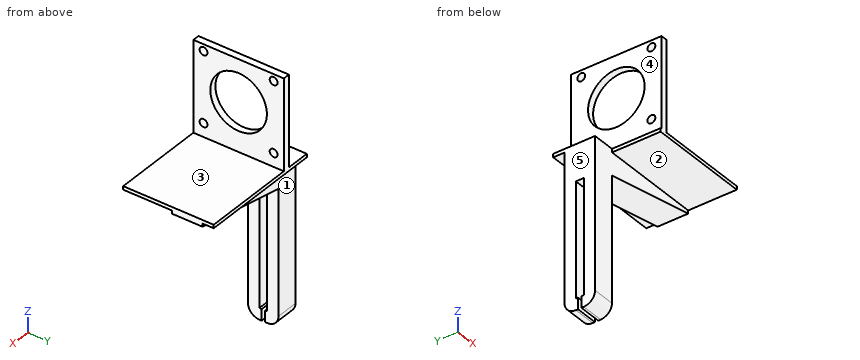
```python
from build123d import *

# Parameters (mm, degrees)
F1_DEPTH      = 10
F2_W          = 1.5
F2_H          = 5
F3_DEPTH      = 11
F4_W          = 3
F4_H          = 40
F5_DEPTH      = 35
F5_DEPTH_BACK = 5
F6_W          = 13.5
F6_H          = 10
F7_DEPTH      = 45
F9_DEPTH      = 15
F10_R         = 1.75
F10_R_2       = 12.5
F11_DEPTH     = 25
F12_W         = 10
F12_H         = 21.5
F13_DEPTH     = 25


with BuildPart() as f1:
    # F0 (on Right) → F1 (new body)
    with BuildSketch(Plane.YZ):
        with BuildLine():
            Line((-8.5, 0), (-5, 0))
            ThreePointArc((-5, 0), (-1.464466, 1.464466), (0, 5))
            Line((0, 5), (0, 70))
            Line((0, 70), (-13.5, 70))
            Line((-13.5, 70), (-13.5, 5))
            ThreePointArc((-13.5, 5), (-12.035534, 1.464466), (-8.5, 0))
        make_face()
    extrude(amount=F1_DEPTH)

    # F2 (on face) → F3 (cut)
    with BuildSketch(Plane.YZ.offset(10)):
        Polygon((-5, 55.5), (-8.5, 55.5), (-8.5, 5), (-7.441577, 5), (-5.941577, 5), (-5, 5), align=None)
        with Locations((-6.691577, 2.5)):
            Rectangle(F2_W, F2_H)
    extrude(amount=-F3_DEPTH, mode=Mode.SUBTRACT)

    # F4 (on Front) → F5 (join, two sides)
    with BuildSketch(Plane.XZ) as f5_sk:
        Polygon((10.552509, 71.532604), (0, 71.532604), (0, 70), (55, 70), (55, 71.532604), (13.552509, 71.532604), align=None)
        with Locations((12.052509, 91.532604)):
            Rectangle(F4_W, F4_H)
    extrude(amount=F5_DEPTH)
    extrude(f5_sk.sketch, amount=-F5_DEPTH_BACK)

    # F6 (on face) → F7 (join, through all)
    with BuildSketch(Plane.YZ.offset(10)):
        with Locations((-6.75, 65)):
            Rectangle(F6_W, F6_H)
    extrude(amount=F7_DEPTH)

    # F8 (on face) → F9 (cut)
    with BuildSketch(Plane.XZ.offset(13.5)):
        Polygon((55, 68.611123), (10, 60), (55, 60), align=None)
    extrude(amount=-F9_DEPTH, mode=Mode.SUBTRACT)

    # F10 (on face) → F11 (cut)
    with BuildSketch(Plane(origin=(10.552509, 0, 0), x_dir=(0, -1, 0), z_dir=(-1, 0, 0))):
        with Locations((-0.5, 108.532604)):
            Circle(F10_R)
        with Locations((30.5, 108.532604)):
            Circle(F10_R)
        with Locations((30.5, 77.532604)):
            Circle(F10_R)
        with Locations((-0.5, 77.532604)):
            Circle(F10_R)
        with Locations((15, 93.032604)):
            Circle(F10_R_2)
    extrude(amount=-F11_DEPTH, mode=Mode.SUBTRACT)

    # F12 (on face) → F13 (cut)
    with BuildSketch(Plane.XY.offset(71.532604)):
        with Locations((5, -24.25)):
            Rectangle(F12_W, F12_H)
    extrude(amount=-F13_DEPTH, mode=Mode.SUBTRACT)


solid = f1.part
```
Check sheet for the modelled part. Datum: model origin and axes. Units: mm. Face numbers are marked on the shaded views. A direction names the side the tool comes from. Give positions to 0.01 mm unless a question says otherwise; leave off trailing zeros. Write each loop counter-clockwise with the first axis right and the second up, starting at its lowest first coordinate (ties: lowest second). Pieces come first, ordered by that corner, then holes. Notation, with made-up numbers: (11, -12) -> (18, -12) arc R27 cw to (18, 21) -> close; hole circle Ø1 at (72, 6). An arc over 180 degrees is marked (long way). Use CSV: the item, a comma, the result in double quotes. Start each with the question number.
Q1. Tool access check on the marked faces 1, 2, 3, 4 and 5. Record the directions out of +Z, -Z, +X, -X, +Y, -Y that give a thin tool (end or side, any length) a straight path to the whole face; none if there is none.
Q2. Cross-section at B-B on z = 29. Enter the section's corners in (x, y), and give its area (3 significant figures).
Q3. Cross-section at D-D on x = 4.5. Enter the section's corners in (y, z).
Q4. Cross-section at A-A on y = -15. Enter the section's corners in (x, z).
Q5. Depth check by flat-ended pin: P1, Ø3, axis at x = 29, y = -5, coming from the +Z side; P2, Ø3, axis at y = -30.5, z = 77.53, coming from the +X side; P3, Ø1.2, axis at y = -22, z = 71, coming from the -X side; P4, Ø2.5, axis at x = 5, z = 3, coming from the -Y side. Enter the tip coordinate at first touch or a pass-through.
Q6. Scan lines: line 1 along Z through (x, y) = (12.1, -30.5); line 2 along Z through (x, y) = (11, -30); line 3 along Z through (x, y) = (15, -18). Record each from-to range of solid material in increasing order.
Q7. Cross-section at C-C on y = -30.5. Enter the section's corners in (x, z), and give its area (3 significant figures).
Working result:
1,face 1,"-Z, +X, -X, +Y"
1,face 2,"-Z, +X, -X, -Y"
1,face 3,"+Z, +X, +Y, -Y"
1,face 4,"+Z, -X, +Y, -Y"
1,face 5,"+Z, -Z, -X, +Y, -Y"
2,outline,"(0, -13.5) -> (10, -13.5) -> (10, -8.5) -> (0, -8.5) -> close; (0, -5) -> (10, -5) -> (10, 0) -> (0, 0) -> close"
2,area,"100 mm^2"
3,outline,"(-13.5, 5) arc R5 ccw to (-8.5, 0) -> (-7.44, 0) -> (-7.44, 5) -> (-8.5, 5) -> (-8.5, 55.5) -> (-5, 55.5) -> (-5, 5) -> (-5.94, 5) -> (-5.94, 0) -> (-5, 0) arc R5 ccw to (0, 5) -> (0, 70) -> (5, 70) -> (5, 71.53) -> (-13.5, 71.53) -> close"
4,outline,"(10, 70) -> (55, 70) -> (55, 71.53) -> (13.55, 71.53) -> (13.55, 80.53) -> (10.55, 80.53) -> (10.55, 71.53) -> (10, 71.53) -> close; (10.55, 105.53) -> (13.55, 105.53) -> (13.55, 111.53) -> (10.55, 111.53) -> close"
5,P1,"stops at z = 71.53"
5,P2,"passes through"
5,P3,"stops at x = 10"
5,P4,"stops at y = -13.44"
6,line 1,"z = 70 to 75.78, 79.28 to 106.78, 110.28 to 111.53"
6,line 2,"z = 70 to 75.86, 79.21 to 106.86, 110.21 to 111.53"
6,line 3,"z = 70 to 71.53"
7,outline,"(10, 70) -> (55, 70) -> (55, 71.53) -> (13.55, 71.53) -> (13.55, 75.78) -> (10.55, 75.78) -> (10.55, 71.53) -> (10, 71.53) -> close; (10.55, 79.28) -> (13.55, 79.28) -> (13.55, 106.78) -> (10.55, 106.78) -> close; (10.55, 110.28) -> (13.55, 110.28) -> (13.55, 111.53) -> (10.55, 111.53) -> close"
7,area,"168 mm^2"
